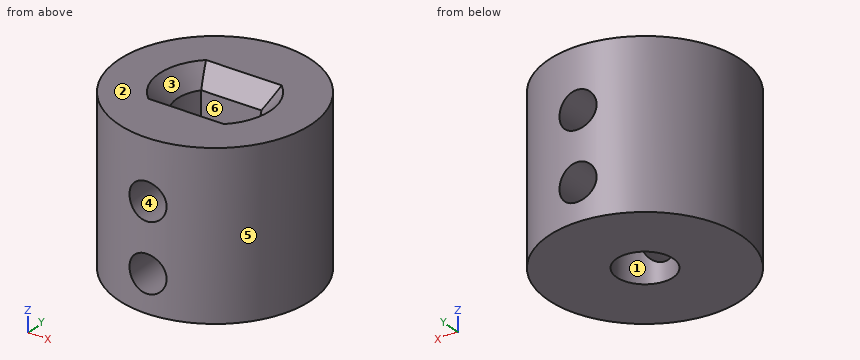
Autodesk Inventor part; units mm, degrees
ref_plane "Work Plane1" through (-20.8033, -6.3, -5.9) normal (0, 0, 1) x (1, 0, 0)
ref_plane "YZ Plane" through (0, 0, 0) normal (1, 0, 0) x (0, 1, 0)
ref_plane "XZ Plane" through (0, 0, 0) normal (0, 1, 0) x (-1, 0, 0)
sketch "Sketch1" plane through (0, 0, 0) normal (0, 0, 1) x (1, 0, 0)
  line L0 (0.8467, -0.7217) -> (0.8467, 0.7217) construction
  line L1 (0.8467, 0.7217) -> (2.0967, 1.4434) construction
  line L2 (2.0967, 1.4434) -> (3.3467, 0.7217) construction
  line L3 (3.3467, 0.7217) -> (3.3467, -0.7217) construction
  line L4 (3.3467, -0.7217) -> (2.0967, -1.4434) construction
  line L5 (2.0967, -1.4434) -> (0.8467, -0.7217) construction
  circle A0 centre (2.0967, 0) radius 2.45 construction
  line L6 (4.8467, -1.5877) -> (3.4717, -2.3816) construction
  line L7 (15.0967, 3) -> (15.0967, -3) construction
  line L8 (-10.9033, 3) -> (-10.9033, -3) construction
  line L9 (-0.6533, 0) -> (-0.6533, 1.5877) construction
  circle A1 centre (2.0967, 0) radius 5
  circle A2 centre (2.0967, 0) radius 1.7
  line L10 (-10.9033, -3) -> (15.0967, -3)
  line L11 (-10.9033, 3) -> (15.0967, 3)
  circle A3 centre (2.0967, 0) radius 1.9
  circle A4 centre (2.0967, 0) radius 6.5
  point P0 (0.4719, -0.5)
  point P1 (3.7215, -0.5)
  dimension "d10" = 3.8
  dimension "d13" = 13
ref_plane "Work Plane1" through (-20.8033, -6.3, -5.9) normal (0, 0, 1) x (1, 0, 0)
extrude "Extrusion1" add sketch "Sketch1" against normal blind 5 contours A1 L10 L11 | A1 L11 A4 L10 | L11 A1 | A1 L11 A4 | L10 A4 A1 | A1 L10 | A1 L10 A4 L11
sketch "Sketch2" plane through (2.0967, 0, 0) normal (0, 0, 1) x (1, 0, 0)
  line L0 (-2, 1.5) -> (2, 1.5) construction
  arc A0 (2.5, 0) -> (2, 1.5) centre (0, 0) ccw construction
  arc A1 (-2, 1.5) -> (-2.5, 0) centre (0, 0) ccw construction
  line L1 (2, -1.5) -> (-2, -1.5) construction
  arc A2 (-2.5, 0) -> (2.5, 0) centre (0, 0) ccw construction
  line L2 (2.0248, 1.55) -> (-2.0248, 1.55) construction
  arc A3 (-2.0248, 1.55) -> (-2.55, 0) centre (0, 0) ccw construction
  arc A4 (-2.55, 0) -> (2.55, 0) centre (0, 0) ccw construction
  arc A5 (2.55, 0) -> (2.0248, 1.55) centre (0, 0) ccw construction
  line L3 (-2.0248, 1.55) -> (2.0248, 1.55) construction
  line L4 (-2.0248, 1.55) -> (2.0248, 1.55)
  line L5 (-2.0248, -1.55) -> (2.0248, -1.55)
  arc A6 (-2.0248, 1.55) -> (-2.0248, -1.55) centre (0, 0) ccw
  arc A7 (2.0248, -1.55) -> (2.0248, 1.55) centre (0, 0) ccw
  circle A8 centre (0, 0) radius 6.5
  point P0 (-2.0967, 0)
  dimension "d11" = 3.1
  dimension "d12" = 2.55
extrude "Extrusion2" add sketch "Sketch2" along normal blind 6
chamfer "Chamfer1" distance 1.2 angle 45 4 edges at (2.0967, 1.55, 6) (-0.4533, 0, 6) (2.0967, -1.55, 6) (4.6467, 0, 6)
sketch "Sketch3" plane through (0, 0, 0) normal (0, 1, 0) x (-1, 0, 0)
  line L0 (-4.6467, 0) -> (-4.6467, 4.8)
  line L1 (0.4533, 0) -> (0.4533, 4.8)
  line L2 (-8.5967, -5) -> (4.4033, -5)
  circle A0 centre (-2.0967, -2.5) radius 1.25
  line L3 (-8.5967, -5) -> (4.4033, -5)
  point P0 (0, 0)
  point P1 (-8.5967, 0)
  point P2 (4.4033, 0)
  dimension "d14" = 2.5
  dimension "d15" = 2.5
extrude "Extrusion3" cut sketch "Sketch3" against normal blind 10
pattern_circular "Circular Pattern1" count 2 over 360 about axis through (2.0967, 0, 0) along (0, 0, -1) of "Extrusion3"
sketch "Sketch4" plane through (0.0718, -1.55, 0) normal (0, 1, 0) x (1, 0, 0)
  line L0 (0, -4.8) -> (4.0497, -4.8)
  line L1 (-4.4752, -6) -> (8.5248, -6)
  line L2 (8.5248, 5) -> (-4.4752, 5)
  line L3 (4.0497, -4.8) -> (0, -4.8)
  line L4 (4.0497, 0) -> (4.0497, -4.8)
  line L5 (0.926, 0) -> (3.1237, 0)
  line L6 (0, 0) -> (0, -4.8)
  circle A0 centre (2.0248, -2.0248) radius 2.0248
  line L7 (3.1237, 0) -> (4.0497, 0)
  line L8 (0, 0) -> (0.926, 0)
  point P0 (-0.0718, 0)
  point P1 (3.2748, 2.5)
  point P2 (0.7748, 2.5)
hole "Hole1" at (2.0967, -1.55, 2.0248) direction (0, -1, 0) diameter 2.5 end through all both
properties part number "30_Coupling_Screw_28BYJ_M4_v2"
Can you work these out from the model? Positions are in its coordinate system, mm. Face numbers are marked on the shaded views. A direction names the side the tool comes from. Give positions to 0.01 mm unless a question says otherwise; leave off trailing zeros. Write each loop counter-clockwise with the first axis right and the second up, starting at its lowest first coordinate (ties: lowest second). Pieces come first, ordered by that corner, then holes. Notation, with made-up numbers: (13, 87.5) -> (26, 87.5) arc R24 cw to (26, 99.5) -> close; hole circle Ø4 at (44, 28). An arc over 180 degrees is marked (long way). One line per item, written item: value.
Q1. We'd pull the mould along Y, two halves only. Please class the marked faces 4, 5 and 6: +Y half, -Y half, draft (parallel to the pull), parting line (faces both ways), or undercut.
Results found:
face 4: draft
face 5: parting line
face 6: undercut
Q2. Imagine slicing it at C-C on x = 1.75. Give the number of separate pieces and of enclosed holes in the cut face, and give its area (3 significant figures).
Results found:
separate pieces: 6
enclosed holes: 0
area: 58.1 mm^2
Q3. Imagine slicing it at A-A on y = 0. Please give me the cut outline in (x, z).
Results found:
outline: (-4.4, -5) -> (0.2, -5) -> (0.2, 0) -> (-0.45, 0) -> (-0.45, 4.8) -> (-1.65, 6) -> (-4.4, 6) -> close; (4, -5) -> (8.6, -5) -> (8.6, 6) -> (5.85, 6) -> (4.65, 4.8) -> (4.65, 0) -> (4, 0) -> close
Q4. Imagine slicing it at D-D on z = -2.5. Please give me the cut outline in (x, y), and give its area (3 significant figures).
Results found:
outline: (0.85, -6.38) -> (0.85, -1.43) arc R1.9 cw to (0.85, 1.43) -> (0.85, 6.38) arc R6.5 ccw to start; (3.35, -6.38) arc R6.5 ccw to (3.35, 6.38) -> (3.35, 1.43) arc R1.9 cw to (3.35, -1.43) -> close
area: 97.9 mm^2
Q5. Imagine slicing it at B-B on z = 2.75. Please give me the cut outline in (x, y), and give its area (3 significant figures).
Results found:
outline: (0.07, -1.55) arc R2.55 cw to (0.07, 1.55) -> (1.08, 1.55) -> (1.08, 6.42) arc R6.5 ccw to (1.08, -6.42) -> (1.08, -1.55) -> close; (3.11, -6.42) arc R6.5 ccw to (3.11, 6.42) -> (3.11, 1.55) -> (4.12, 1.55) arc R2.55 cw to (4.12, -1.55) -> (3.11, -1.55) -> close
area: 97.9 mm^2
Q6. Please list where these lines run through material, in increasing order: line 1 (Z direction, x = 2, y = -2.5); line 2 (Z direction, x = 1.25, y = 5.5); line 3 (X direction, y = -0.25, z = -1). Write a range as [from, to].
Results found:
line 1: z = [-5, -3.75], [-1.25, 0.78], [3.27, 5.75]
line 2: z = [-5, -3.42], [-1.58, 1.11], [2.94, 6]
line 3: x = [-4.4, 0.21], [3.98, 8.59]
Q7. For P1, Ø5, axis at x = 1.5, z = 3.5, coming from the -Y side; P2, Ø1.6, axis at x = 4, y = 0.5, coming from the +Z side; P3, Ø4, axis at x = -3, z = 4, coming from the -Y side; P4, Ø1.5, axis at y = 4, z = -1.5, coming from the +X side, each with a flat end and sliding along its axis, tell me the tip position at first contact or that it passes through.
Results found:
P1: stops at y = -6.5
P2: stops at z = 5.02
P3: stops at y = -5.71
P4: stops at x = 7.73
Q8. Which directions (+Z, -Z, +X, -X, +Y, -Y) give clear straight access to the entire face, cutting with the end or side of a thin tool? Please do the marked faces 1, 2 and 3.
Results found:
face 1: -Z
face 2: +Z, +X, -X, +Y, -Y
face 3: +Z
